from build123d import *

# Parameters (mm, degrees)
F0_W      = 1000
F0_H      = 150
F1_DEPTH  = 1800
F5_DEPTH  = 250
F7_DEPTH  = 250
F8_W      = 1814.4553899765
F8_H      = 676.3893961906
F9_DEPTH  = 500
F10_DEPTH = 500
F11_W     = 1876.0774359107
F11_H     = 584.96324718
F12_DEPTH = 490


# Not quite as in the source:
# - the dataset's text gives a spline's control points without its knots; the knots are read off the source's solid


with BuildPart() as f1:
    # F0 (on Front) → F1 (new body)
    with BuildSketch(Plane.XZ):
        with Locations((427.8578534722, -75)):
            Rectangle(F0_W, F0_H)
    extrude(amount=F1_DEPTH)

    # F4 (on plane+point) → F5 (join, symmetric)
    with BuildSketch(Plane.YZ.offset(427.8578534722)):
        with BuildLine():
            add(Edge.make_bspline(
                [(-658.5119275224, 0), (-663.1096709351, -3.3994040102), (-674.8923410513, -12.2269214906), (-701.8084297627, -13.9660228128), (-718.060195446, -15.0110442191)],
                knots=[0, 0, 0, 0, 0.3960668718, 1, 1, 1, 1], degree=3))
            add(Edge.make_bspline(
                [(-658.5119275224, 0), (-650.3595915647, 6.0275402647), (-648.0235359943, 31.4958112046), (-617.163744576, 46.1983191108), (-607.3494242193, 51.7760817812)],
                knots=[0, 0, 0, 0, 0.4646733695, 1, 1, 1, 1], degree=3))
            Line((-607.3494242193, 51.7760817812), (-607.3494242193, 331.3955929823))
            ThreePointArc((-607.3494242193, 331.3955929823), (-611.1459562468, 329.3507401392), (-613.7284624486, 325.8973736217))
            Line((-613.7284624486, 325.8973736217), (-746.2776173449, 32.8608466306))
            ThreePointArc((-746.2776173449, 32.8608466306), (-751.7911260188, 25.6605897485), (-759.9176837495, 21.6354765186))
            Line((-759.9176837495, 21.6354765186), (-851.8334031105, 0))
            Line((-851.8334031105, 0), (-724.4437932968, 0))
            Line((-724.4437932968, 0), (-718.060195446, -15.0110442191))
        make_face()
    extrude(amount=F5_DEPTH, both=True)

    # F6 (on plane+point) → F7 (cut, symmetric)
    with BuildSketch(Plane.YZ.offset(427.8578534722)):
        with BuildLine():
            add(Edge.make_bspline(
                [(-657.9174152342, -0.8040865247), (-659.3673865445, -1.8761424975), (-662.3030933204, -4.0564869069), (-666.4204873665, -6.6707717939), (-670.1931092733, -8.5651184529), (-673.3105086069, -9.8565410415), (-676.7740170416, -10.9816784698), (-681.8145421149, -12.2587633506), (-688.8193216778, -13.5004768766), (-698.0763714753, -14.5692911085), (-707.8993120937, -15.3593398489), (-714.632248917, -15.792685566), (-717.9960259489, -16.0089832331)],
                knots=[0, 0, 0, 0, 0.125, 0.25, 0.3125, 0.375, 0.4375, 0.5, 0.625, 0.75, 0.875, 1, 1, 1, 1], degree=3))
            Line((-657.9174152342, -0.8040865247), (-656.8298765035, 0))
            Line((-656.8298765035, 0), (-658.5119275224, 0))
            add(Edge.make_bspline(
                [(-658.5119275224, 0), (-663.1096709351, -3.3994040102), (-674.8923410513, -12.2269214906), (-701.8084297627, -13.9660228128), (-718.060195446, -15.0110442191)],
                knots=[0, 0, 0, 0, 0.3960668718, 1, 1, 1, 1], degree=3))
            Line((-718.060195446, -15.0110442191), (-717.9960259489, -16.0089832331))
        make_face()
    extrude(amount=F7_DEPTH, both=True, mode=Mode.SUBTRACT)

    # F8 (on plane+point) → F9 (cut, through all)
    with BuildSketch(Plane.YZ.offset(427.8578534722)):
        with Locations((-907.2276949883, 182.6078593731)):
            Rectangle(F8_W, F8_H)
    extrude(amount=F9_DEPTH, mode=Mode.SUBTRACT)

    # F10 (add): a face of the model
    f10_faces = [f1.faces().sort_by_distance(p)[0] for p in [
        (302.8578534722, -607.3494242193, 191.5858373818),
    ]]
    extrude(f10_faces, amount=F10_DEPTH)

    # F11 (on face) → F12 (cut)
    with BuildSketch(Plane(origin=(-72.1421465278, 0, 0), x_dir=(0, -1, 0), z_dir=(-1, 0, 0))):
        with Locations((910.4874022305, 71.823425591)):
            Rectangle(F11_W, F11_H)
    extrude(amount=-F12_DEPTH, mode=Mode.SUBTRACT)


solid = f1.part
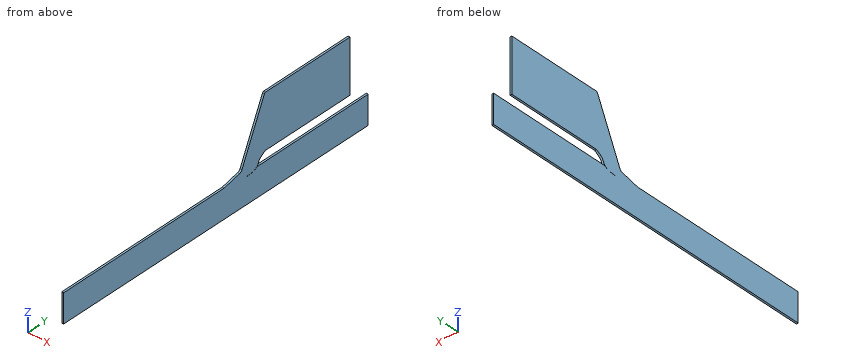
CAD build for the part. Positions are in the model's coordinates, mm. Give positions to 0.01 mm unless a question says otherwise; leave off trailing zeros. Write each loop counter-clockwise with the first axis right and the second up, starting at its lowest first coordinate (ties: lowest second). Pieces come first, ordered by that corner, then holes. Notation, with made-up numbers: M 6.5,38 L 53.5,38 A13 cw 53.5,47 Z; hole C -23,3 d1. An arc over 180 degrees is marked long. Put each result on its own line as item: value. Start each with the question number.
(1) Band-saw the part on B-B, the plane y = -1042.5. Write the cut outline in (x, z).
(2) Band-saw the part on A-A, the plane y = -356.5. Write the cut outline in (x, z), and give its area (3 significant figures).
(3) Band-saw the part on C-C, the plane z = 75. Write the cut outline in (x, y), and give its area (3 significant figures).
(4) Probe L1, parallel to Z at x = 423.75, y = -484; L2, parallel to Y at x = 424.5, z = 303; L3, parallel to Y at x = 424.25, z = -7. List the from-to ranges inside material, lowest first.
(5) Flat gauge pins, fed straight in: pin 1 Ø5 at (x, y) = (424.5, -1258) entering from +Z; pin 2 Ø1 at (x, z) = (419, 115.5) entering from -Y; pin 3 Ø2 at (x, z) = (420.5, 130) entering from -Y. Where does each tip first touch, or does it go through?
Response values:
1. outline: M 417.86,-150 L 427.86,-150 L 427.86,0 L 417.86,0 Z
2. outline: M 417.86,-150 L 427.86,-150 L 427.86,0 L 417.86,0 Z; M 417.86,51.78 L 427.86,51.78 L 427.86,331.4 L 417.86,331.4 Z
2. area: 4,300 mm2
3. outline: M 417.86,-727.22 L 427.86,-727.22 L 427.86,-107.35 L 417.86,-107.35 Z
3. area: 6,200 mm2
4. L1: z = -150 to 0, 51.78 to 331.4
4. L2: y = -624.09 to -107.35
4. L3: y = -1800 to -669.33, -667.17 to 0
5. pin 1: stops at z = 0
5. pin 2: stops at y = -709.12
5. pin 3: stops at y = -702.79
